from build123d import *

# Parameters (mm, degrees)
BASEPLATE_OUTLINE_R = 2.1
BASEPLATE_DEPTH     = 2.8
CUT_EXTRUDE1_REACH  = 115.438
FILLET1_R           = 1


# Read off the part's stored shape, not the designer's step: BasePlate
with BuildPart() as part:
    # BasePlate outline → BasePlate (new body)
    with BuildSketch(Plane(origin=(0, 0, 0), x_dir=(1, 0, 0), z_dir=(0, 1, 0))):
        with BuildLine():
            Line((43.502626614, -5.852332608), (48.792614178, -5.852332608))
            ThreePointArc((48.792614178, -5.852332608), (49.082078508, -5.760021707), (49.264659986, -5.517174213))
            Line((49.264659986, -5.517174213), (50.078201202, -3.187491002))
            ThreePointArc((50.078201202, -3.187491002), (50.26078268, -2.944643509), (50.55024701, -2.852332608))
            Line((50.55024701, -2.852332608), (58.116695703, -2.852332608))
            ThreePointArc((58.116695703, -2.852332608), (58.484685739, -3.013831008), (58.614956567, -3.393999275))
            ThreePointArc((58.614956567, -3.393999275), (64.799237397, -7.61016844), (65.229166667, -0.137781095))
            ThreePointArc((65.229166667, -0.137781095), (65.061014427, 0.043158816), (65, 0.282515593))
            Line((65, 0.282515593), (65, 83.012819192))
            ThreePointArc((65, 83.012819192), (65.061014427, 83.252175969), (65.229166667, 83.433115879))
            ThreePointArc((65.229166667, 83.433115879), (65.940559159, 90.088226551), (59.285448487, 89.376834059))
            ThreePointArc((59.285448487, 89.376834059), (59.104508577, 89.208681819), (58.8651518, 89.147667392))
            Line((58.8651518, 89.147667392), (6.1348482, 89.147667392))
            ThreePointArc((6.1348482, 89.147667392), (5.895491423, 89.208681819), (5.714551513, 89.376834059))
            ThreePointArc((5.714551513, 89.376834059), (-0.940559159, 90.088226551), (-0.229166667, 83.433115879))
            ThreePointArc((-0.229166667, 83.433115879), (-0.061014427, 83.252175969), (0, 83.012819192))
            Line((0, 83.012819192), (0, 0.282515593))
            ThreePointArc((0, 0.282515593), (-0.061014427, 0.043158816), (-0.229166667, -0.137781095))
            ThreePointArc((-0.229166667, -0.137781095), (0.200762603, -7.61016844), (6.385043433, -3.393999275))
            ThreePointArc((6.385043433, -3.393999275), (6.515314261, -3.013831008), (6.883304297, -2.852332608))
            Line((6.883304297, -2.852332608), (14.44975299, -2.852332608))
            ThreePointArc((14.44975299, -2.852332608), (14.73921732, -2.944643509), (14.921798798, -3.187491002))
            Line((14.921798798, -3.187491002), (15.735340014, -5.517174213))
            ThreePointArc((15.735340014, -5.517174213), (15.917921492, -5.760021707), (16.207385822, -5.852332608))
            Line((16.207385822, -5.852332608), (21.497373386, -5.852332608))
            ThreePointArc((21.497373386, -5.852332608), (21.786837716, -5.760021707), (21.969419194, -5.517174213))
            Line((21.969419194, -5.517174213), (22.78296041, -3.187491002))
            ThreePointArc((22.78296041, -3.187491002), (22.965541888, -2.944643509), (23.255006218, -2.852332608))
            Line((23.255006218, -2.852332608), (41.744993782, -2.852332608))
            ThreePointArc((41.744993782, -2.852332608), (42.034458112, -2.944643509), (42.21703959, -3.187491002))
            Line((42.21703959, -3.187491002), (43.030580806, -5.517174213))
            ThreePointArc((43.030580806, -5.517174213), (43.213162284, -5.760021707), (43.502626614, -5.852332608))
        make_face()
        with Locations((2.1, -3.752332608)):
            Circle(BASEPLATE_OUTLINE_R, mode=Mode.SUBTRACT)
        with Locations((62.9, -3.752332608)):
            Circle(BASEPLATE_OUTLINE_R, mode=Mode.SUBTRACT)
        with Locations((2.1, 87.047667392)):
            Circle(BASEPLATE_OUTLINE_R, mode=Mode.SUBTRACT)
        with Locations((62.9, 87.047667392)):
            Circle(BASEPLATE_OUTLINE_R, mode=Mode.SUBTRACT)
    extrude(amount=BASEPLATE_DEPTH)

    # Sketch3 → Cut-Extrude1 (cut, up to next)
    with BuildSketch(Plane(origin=(0, 2.8, 0), x_dir=(1, 0, 0), z_dir=(0, 1, 0)), mode=Mode.PRIVATE) as cut_extrude1_sk1:
        Polygon((6, 83.647667392), (6, 4.347667392), (22.9, 4.347667392), (22.9, -3.00023804), (42.1, -3.00023804), (42.1, 4.347667392), (61.3, 4.347667392), (61.3, 83.647667392), align=None)
    cut_extrude1_tool1 = extrude(cut_extrude1_sk1.sketch, amount=-CUT_EXTRUDE1_REACH, mode=Mode.PRIVATE) & part.part
    add(cut_extrude1_tool1.solids().sort_by_distance((33.614156, 2.8, -42.647328))[0], mode=Mode.SUBTRACT)

    # Fillet1
    fillet1_edges = [part.edges().sort_by_distance(p)[0] for p in [
        (6, 1.4, -83.647667392),
        (61.3, 1.4, -83.647667392),
        (61.3, 1.4, -4.347667392),
        (6, 1.4, -4.347667392),
    ]]
    fillet(fillet1_edges, radius=FILLET1_R)


solid = part.part
Could you check a few things on this model? Use its own coordinates, in mm. A direction names the side the tool comes from. Give positions to 0.01 mm unless a question says otherwise; leave off trailing zeros. Order: outer loops, then holes, each group sorted by start corner. A loop starts at its lowest first (then second) coordinate and runs counter-clockwise, first axis right, second up.
Item 1: I need wall thicknesses on line 1 (Z direction, x = 62.9, y = 0.8); line 2 (X direction, y = 2.2, z = -47.5); line 3 (X direction, y = 1.8, z = 4). Which ranges of each line are inside material? Lowest first, please.
Item 2: If we section it at A-A, the plane x = 45: Write out the boundary of the cut face in (y, z).
Item 3: If we mould it in two halves opening along Z, with no side actions, what happens to faces 4 (the face through (42.62, 1.38, 4.34)), 5 (the face through (33, 1, -89.148)), 6 (the face through (65, 1, -41))? For each: pulls with the +Z half, pulls with the -Z half, needs draft (parallel to the pull), parting line crosses it, or undercut.
Item 4: If we section it at C-C, the plane x = 62.9: Write out the boundary of the cut face in (y, z), plus the area to 3 significant figures.
Item 5: I'm going to push flat-ended pins straight in: pin 1 (0.8 mm diameter, centred on x = 9.5, y = 1, fed in from +Z); pin 2 (1.4 mm diameter, centred on y = 1.5, z = -24, fed in from -X); pin 3 (1.4 mm diameter, centred on x = 45, y = 1.5, fed in from +Z); pin 4 (4 mm diameter, centred on x = 62.9, z = -87.05, fed in from -Y). Where does each tip first touch, or does it pass through?
Item 6: For faces 1 (the face through (34, 1, -83.648)), 2 (the face through (0, 1, -42)), 3 (the face through (22.37, 1.38, 4.37)), which set-ups out of +Z, -Z, +X, -X, +Y, -Y let a thin tool reach every point of the face, with its end or its side?
Item 7: If we section it at B-B, the plane z = -43: Write out the boundary of the cut face in (x, y), plus the area to 3 significant figures.
Item 8: If we section it at D-D, the plane y = 1.7: Count the separate pieces of the cut face and the enclosed holes in it, plus the area to 3 significant figures.
Values:
1. line 1: z = -91.35 to -89.15, -84.95 to 1.65, 5.85 to 8.05
1. line 2: x = 0 to 6, 61.3 to 65
1. line 3: x = -2.19 to 0.01, 4.19 to 6.39, 15.21 to 22.5, 42.5 to 49.79, 58.61 to 60.81, 64.99 to 67.19
2. outline: (0, -89.15) - (2.8, -89.15) - (2.8, -83.65) - (0, -83.65) - close; (0, -4.35) - (2.8, -4.35) - (2.8, 5.85) - (0, 5.85) - close
3. face 4: pulls with the +Z half
3. face 5: pulls with the -Z half
3. face 6: undercut
4. outline: (0, -91.35) - (2.8, -91.35) - (2.8, -89.15) - (0, -89.15) - close; (0, -84.95) - (2.8, -84.95) - (2.8, 1.65) - (0, 1.65) - close; (0, 5.85) - (2.8, 5.85) - (2.8, 8.05) - (0, 8.05) - close
4. area: 255 mm2
5. pin 1: stops at z = 2.85
5. pin 2: stops at x = 0
5. pin 3: stops at z = 5.85
5. pin 4: passes through
6. face 1: +Y, -Y
6. face 2: -X, +Y, -Y
6. face 3: +Z, +Y, -Y
7. outline: (0, 0) - (6, 0) - (6, 2.8) - (0, 2.8) - close; (61.3, 0) - (65, 0) - (65, 2.8) - (61.3, 2.8) - close
7. area: 27.2 mm2
8. separate pieces: 1
8. enclosed holes: 4
8. area: 1,570 mm2
